Could you check a few things on this model? Use its own coordinates, in mm. A direction names the side the tool comes from. Round coordinates to 2 decimals unless told otherwise and drop trailing zeros. Loops run counter-clockwise (first coordinate to the right, second up) from the corner with the lowest first, then second, coordinate; pieces in that order, holes last. Notation, with made-up numbers: (58, 84.5) -> (64, 84.5) arc R13 ccw to (64, 104.5) -> close; hole circle Ø6 at (82, 13.25). An arc over 180 degrees is marked (long way). Put each result on its own line as item: value. Start each with the question number.
1. Which directions (+Z, -Z, +X, -X, +Y, -Y) give clear straight access to the entire face, cutting with the end or side of a thin tool? Please do faces 1 (the flat face through (-47, -35, -4.5)), 2 (the flat face through (-46.26, -34.51, 0.06)).
2. Imagine slicing it at A-A, the plane z = 2.25. Please give me the cut outline in (x, y), and give its area (3 significant figures).
3. If we mould it in two halves opening along X, with no side actions, what happens to faces 3 (the flat face through (-29, -48, 4.5)), 4 (the flat face through (-47.49, -33.65, -0.06)), 5 (the cylindrical face through (3.74, 18.49, 0.06)), 6 (the cylindrical face through (-78.89, -99.965, -0.063))? For each: pulls with the +X half, pulls with the -X half, needs draft (parallel to the pull), parting line crosses it, or undercut.
4. Imagine slicing it at C-C, the plane y = -35.5. Please give me the cut outline in (x, z), and give its area (3 significant figures).
5. Imagine slicing it at B-B, the plane x = -35. Please give me the cut outline in (y, z).
6. I'm going to push flat-ended pins straight in: P1, Ø2, axis at y = -54.5, z = -1, coming from the -X side; P2, Ø8, axis at x = -7.5, y = -26.5, coming from the +Z side. Where does each tip first touch, or does it pass through?
7. I need wall thicknesses on line 1 (Y direction, x = -50, z = 1.5); line 2 (Y direction, x = -73.5, z = -3.5); line 3 (X direction, y = 4.5, z = 2). Which ranges of each line are inside material? Lowest first, please. Write a range as [from, to].
```python
from build123d import *

# Parameters (mm, degrees)
SKETCH2_W = 1.5
SKETCH2_H = 9


with BuildPart() as part:
    # Sweep1: sweep along a path in Sketch1
    with BuildLine(Plane.XY) as sweep1_path:
        Line((6.319054119, 1.762345914), (-63.556322052, -97.660180283))
        ThreePointArc((-63.556322052, -97.660180283), (-79.51547051, -100.445491543), (-82.30078177, -84.486343085))
        Line((-82.30078177, -84.486343085), (-12.425405599, 14.936183112))
        ThreePointArc((-12.425405599, 14.936183112), (3.533742859, 17.721494372), (6.319054119, 1.762345914))
    # Sketch2 → Sweep1 (sweep)
    with BuildSketch(Plane(origin=(-12.425405599, 14.936183112, 0), x_dir=(0.818149507, -0.575005552, 0), z_dir=(0.575005552, 0.818149507, 0))):
        Rectangle(SKETCH2_W, SKETCH2_H)
    sweep(path=sweep1_path.line)


solid = part.part
```
Entries:
1. face 1: -Z, +X, -X, +Y, -Y
1. face 2: +Z, -Z
2. outline: (-82.91, -84.06) arc R12.21 ccw to (-62.94, -98.09) -> (6.93, 1.33) arc R12.21 ccw to (-13.04, 15.37) -> close; hole (-81.69, -84.92) arc R10.71 ccw to (-64.17, -97.23) -> (5.71, 2.19) arc R10.71 ccw to (-11.81, 14.5) -> close
2. area: 473 mm^2
3. face 3: needs draft
3. face 4: pulls with the -X half
3. face 5: parting line crosses it
3. face 6: undercut
4. outline: (-48.79, -4.5) -> (-46.96, -4.5) -> (-46.96, 4.5) -> (-48.79, 4.5) -> close; (-20.79, -4.5) -> (-18.95, -4.5) -> (-18.95, 4.5) -> (-20.79, 4.5) -> close
4. area: 33.0 mm^2
5. outline: (-58.33, -4.5) -> (-55.72, -4.5) -> (-55.72, 4.5) -> (-58.33, 4.5) -> close; (-18.49, -4.5) -> (-15.88, -4.5) -> (-15.88, 4.5) -> (-18.49, 4.5) -> close
6. P1: x = -62.85
6. P2: through
7. line 1: [-79.68, -77.07], [-39.83, -37.22]
7. line 2: [-103.27, -101.76], [-73.27, -70.66]
7. line 3: [-20.68, -18.84], [6.94, 8.53]
